Source: CAD feature listing. Evaluate the final solid. Frame: model axes, mm. Face numbers are marked on the shaded views. A direction names the side the tool comes from. Give positions to 0.01 mm unless a question says otherwise; leave off trailing zeros. Order: outer loops, then holes, each group sorted by start corner. A loop starts at its lowest first (then second) coordinate and runs counter-clockwise, first axis right, second up.
1) Section D-D, the plane x = -17. Return loops of the section in (y, z).
2) Section B-B, the plane y = 37.6. Return loops of the section in (x, z).
3) Section C-C, the plane x = -55.5. Return loops of the section in (y, z) (3 decimals).
4) First-contact query: P1, Ø2, axis at y = -18, z = -32.5, coming from the +X side; P2, Ø12, axis at x = -21.5, z = -14.5, coming from the -Y side; P3, Ø2.5, axis at y = 15.5, z = 15.5, coming from the -X side. Flat tips, straight axial feed; report the tip coordinate or a pass-through.
5) Section A-A, the plane x = -7. Return loops of the section in (y, z), plus the area to 3 significant figures.
6) Access query for the marked faces 1, 2 and 3. Directions: +Z, -Z, +X, -X, +Y, -Y. A direction counts if a zero-diameter tool reaches every point of the face in a straight line with its end or side. Return the directions, or none.
7) Draft query along Z for the marked faces 4 and 5. Return one class per face: released by +Z, released by -Z, zero draft, split by the parting line, or undercut.
8) Material intervals for line 1 (Z direction, x = -13.5, y = 15); line 2 (X direction, y = 39, z = -3.5); line 3 (Z direction, x = 0.5, y = 8.5), sorted ascending.
```python
from build123d import *

# Parameters (mm, degrees)
CROQUIS1_R                                           = 32.7
CROQUIS1_R_2                                         = 5
SALIENTE_EXTRUIR1_DEPTH                              = 4.25
REFRENTADO_PARA_TORNILLO_CON_CABEZA_TRON_D           = 3.4
REFRENTADO_PARA_TORNILLO_CON_CABEZA_TRON_CBORE_D     = 7
REFRENTADO_PARA_TORNILLO_CON_CABEZA_TRON_CBORE_DEPTH = 2.4
CROQUIS5_R                                           = 32.7
CROQUIS5_R_2                                         = 21.5
SALIENTE_EXTRUIR2_DEPTH                              = 55
TALADRO_DE_MARGEN_PARA_M31_D                         = 3.4
TALADRO_DE_MARGEN_PARA_M31_DEPTH                     = 15
TALADRO_DE_MARGEN_PARA_M31_TIP                       = 1.021463052
TALADRO_DE_MARGEN_PARA_M32_D                         = 3.4
TALADRO_DE_MARGEN_PARA_M32_DEPTH                     = 16.5
TALADRO_DE_MARGEN_PARA_M32_TIP                       = 1.021463052
CROQUIS16_R                                          = 42.5
SALIENTE_EXTRUIR3_DEPTH                              = 7.5
REFRENTADO_PARA_TORNILLO_CON_CABEZA_2_D              = 3.4
REFRENTADO_PARA_TORNILLO_CON_CABEZA_2_CBORE_D        = 7
REFRENTADO_PARA_TORNILLO_CON_CABEZA_2_CBORE_DEPTH    = 2.4


with BuildPart() as part:
    # Croquis1 → Saliente-Extruir1 (new, symmetric)
    with BuildSketch(Plane(origin=(0, 0, 0), x_dir=(0, 0, -1), z_dir=(1, 0, 0))):
        Circle(CROQUIS1_R)
        Circle(CROQUIS1_R_2, mode=Mode.SUBTRACT)
    extrude(amount=SALIENTE_EXTRUIR1_DEPTH, both=True)

    # Refrentado para tornillo con cabeza tron (through all)
    with Locations(Plane(origin=(4.25, 0, 0), x_dir=(0, 0, -1), z_dir=(1, 0, 0))):
        with Locations((8.838834765, 8.838834765), (-8.838834765, -8.838834765), (-8.838834765, 8.838834765), (8.838834765, -8.838834765)):
            CounterBoreHole(REFRENTADO_PARA_TORNILLO_CON_CABEZA_TRON_D / 2, REFRENTADO_PARA_TORNILLO_CON_CABEZA_TRON_CBORE_D / 2, REFRENTADO_PARA_TORNILLO_CON_CABEZA_TRON_CBORE_DEPTH)

    # Croquis5 → Saliente-Extruir2 (add)
    with BuildSketch(Plane.ZY.offset(4.25)):
        Circle(CROQUIS5_R)
        Circle(CROQUIS5_R_2, mode=Mode.SUBTRACT)
    extrude(amount=SALIENTE_EXTRUIR2_DEPTH)

    # Taladro de margen para M31
    with Locations(Plane.ZY.offset(59.25)):
        with Locations((17.075, 17.075), (-17.075, -17.075), (-17.075, 17.075), (17.075, -17.075)):
            Hole(TALADRO_DE_MARGEN_PARA_M31_D / 2, depth=TALADRO_DE_MARGEN_PARA_M31_DEPTH)
            with Locations((0, 0, -(TALADRO_DE_MARGEN_PARA_M31_DEPTH + TALADRO_DE_MARGEN_PARA_M31_TIP / 2))):  # 118° drill point
                Cone(0, TALADRO_DE_MARGEN_PARA_M31_D / 2, TALADRO_DE_MARGEN_PARA_M31_TIP, mode=Mode.SUBTRACT)

    # Taladro de margen para M32
    with Locations(Plane(origin=(4.25, 0, 0), x_dir=(0, 0, -1), z_dir=(1, 0, 0))):
        with Locations((15.5, 15.5), (-15.5, -15.5), (-15.5, 15.5), (15.5, -15.5)):
            Hole(TALADRO_DE_MARGEN_PARA_M32_D / 2, depth=TALADRO_DE_MARGEN_PARA_M32_DEPTH)
            with Locations((0, 0, -(TALADRO_DE_MARGEN_PARA_M32_DEPTH + TALADRO_DE_MARGEN_PARA_M32_TIP / 2))):  # 118° drill point
                Cone(0, TALADRO_DE_MARGEN_PARA_M32_D / 2, TALADRO_DE_MARGEN_PARA_M32_TIP, mode=Mode.SUBTRACT)

    # Croquis16 → Saliente-Extruir3 (add)
    with BuildSketch(Plane.ZY.offset(59.25)):
        Circle(CROQUIS16_R)
        with BuildLine():
            Line((-18.5, -21.5), (18.5, -21.5))
            ThreePointArc((18.5, -21.5), (20.621320344, -20.621320344), (21.5, -18.5))
            Line((21.5, -18.5), (21.5, 18.5))
            ThreePointArc((21.5, 18.5), (20.621320344, 20.621320344), (18.5, 21.5))
            Line((18.5, 21.5), (-18.5, 21.5))
            ThreePointArc((-18.5, 21.5), (-20.621320344, 20.621320344), (-21.5, 18.5))
            Line((-21.5, 18.5), (-21.5, -18.5))
            ThreePointArc((-21.5, -18.5), (-20.621320344, -20.621320344), (-18.5, -21.5))
        make_face(mode=Mode.SUBTRACT)
    extrude(amount=SALIENTE_EXTRUIR3_DEPTH)

    # Refrentado para tornillo con cabeza  2 (through all)
    with Locations(Plane(origin=(-59.25, 0, 0), x_dir=(0, 0, -1), z_dir=(1, 0, 0))):
        with Locations((-32.562555182, 18.8), (0, 37.6), (32.562555182, 18.8), (32.562555182, -18.8), (0, -37.6), (-32.562555182, -18.8)):
            CounterBoreHole(REFRENTADO_PARA_TORNILLO_CON_CABEZA_2_D / 2, REFRENTADO_PARA_TORNILLO_CON_CABEZA_2_CBORE_D / 2, REFRENTADO_PARA_TORNILLO_CON_CABEZA_2_CBORE_DEPTH)


solid = part.part
```
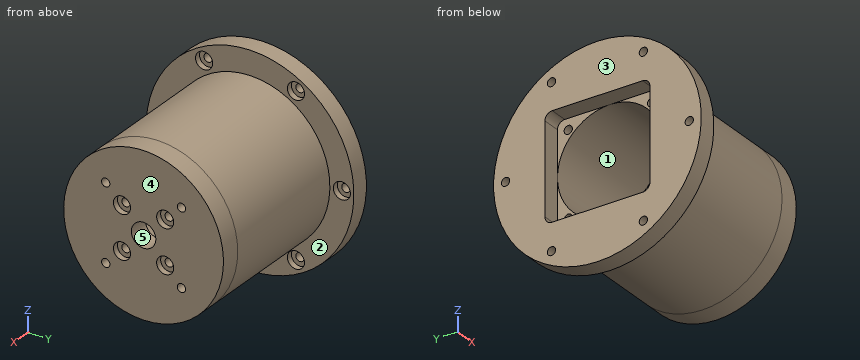
From the geometry:
1. outline: circle Ø65.4 at (0, 0); hole circle Ø43 at (0, 0)
2. outline: (-66.75, -19.81) - (-59.25, -19.81) - (-59.25, -3.5) - (-61.65, -3.5) - (-61.65, -1.7) - (-66.75, -1.7) - close; (-66.75, 1.7) - (-61.65, 1.7) - (-61.65, 3.5) - (-59.25, 3.5) - (-59.25, 19.81) - (-66.75, 19.81) - close
3. outline: circle Ø65.4 at (0, 0); hole circle Ø43 at (0, 0); hole circle Ø3.4 at (-17.075, -17.075); hole circle Ø3.4 at (-17.075, 17.075); hole circle Ø3.4 at (17.075, -17.075); hole circle Ø3.4 at (17.075, 17.075)
4. P1: stops at x = -61.65
4. P2: stops at y = -31.58
4. P3: stops at x = -59.25
5. outline: circle Ø65.4 at (0, 0); hole (-16.31, -14.01) arc R1.7 ccw (long way) to (-14.01, -16.31) arc R21.5 ccw to (14.01, -16.31) arc R1.7 ccw (long way) to (16.31, -14.01) arc R21.5 ccw to (16.31, 14.01) arc R1.7 ccw (long way) to (14.01, 16.31) arc R21.5 ccw to (-14.01, 16.31) arc R1.7 ccw (long way) to (-16.31, 14.01) arc R21.5 ccw to start
5. area: 1,880 mm2
6. face 1: -X
6. face 2: +X
6. face 3: +Z, -Z, -X, +Y, -Y
7. face 4: zero draft
7. face 5: undercut
8. line 1: z = -29.06 to -15.4, 15.4 to 29.06
8. line 2: x = -66.75 to -59.25
8. line 3: z = -31.58 to -10.5, -7.17 to 7.17, 10.5 to 31.58
